Source: CAD feature listing. Evaluate the final solid. Frame: model axes, mm. Round coordinates to 2 decimals unless told otherwise and drop trailing zeros. Loops run counter-clockwise (first coordinate to the right, second up) from the corner with the lowest first, then second, coordinate; pieces in that order, holes last. Notation, with made-up numbers: M -7,78.25 L 30,78.25 A11 cw 30,95.25 Z; hole C 13,57.5 d6. An arc over 180 degrees is marked long. Write each question's results on one line, items separated by ' | '. Start each with the question number.
1. Section B-B on y = -15. Output: boundary loops of the cut face in (x, z).
2. Ray query, line 1 (X direction, y = -3.5, z = -84.5); line 2 (X direction, y = -3, z = -99.5); line 3 (X direction, y = -3, z = -218.5). Return the intervals inside material, ascending.
3. Section A-A on z = -59. Output: boundary loops of the cut face in (x, y).
4. Contact query for flat-ended pins moving along their axis: pin 1 Ø10 at (x, y) = (641.5, -14) entering from +Z; pin 2 Ø1 at (x, y) = (671, -17) entering from +Z; pin 3 Ø10 at (y, z) = (8, -150) entering from -X. Output: stop coordinate, or through.
from build123d import *

# Parameters (mm, degrees)
F0_R     = 25
F1_DEPTH = 1000
F2_R     = 5
F3_DEPTH = 50
F4_R     = 5
F5_DEPTH = 200
F6_R     = 5
F7_DEPTH = 350
F8_R     = 5
F9_DEPTH = 280


with BuildPart() as f1:
    # F0 (on Right) → F1 (new body)
    with BuildSketch(Plane.YZ):
        with Locations((0, 53.862866)):
            Circle(F0_R)
    extrude(amount=F1_DEPTH)

    # F2 (on Top) → F3 (join)
    with BuildSketch(Plane.XY):
        with Locations((500, 0)):
            Circle(F2_R)
        with Locations((250, 0)):
            Circle(F2_R)
        with Locations((750, 0)):
            Circle(F2_R)
    extrude(amount=F3_DEPTH)

    # F4 (on face) → F5 (join)
    with BuildSketch(Plane(origin=(0, 0, 0), x_dir=(1, 0, 0), z_dir=(0, 0, -1))):
        with Locations((750, 0)):
            Circle(F4_R)
    extrude(amount=F5_DEPTH)

    # F6 (on face) → F7 (join)
    with BuildSketch(Plane(origin=(0, 0, 0), x_dir=(1, 0, 0), z_dir=(0, 0, -1))):
        with Locations((500, 0)):
            Circle(F6_R)
    extrude(amount=F7_DEPTH)

    # F8 (on face) → F9 (join)
    with BuildSketch(Plane(origin=(0, 0, 0), x_dir=(1, 0, 0), z_dir=(0, 0, -1))):
        with Locations((250, 0)):
            Circle(F8_R)
    extrude(amount=F9_DEPTH)


solid = f1.part
Taken from the geometry:
1) outline: M 0,33.86 L 1000,33.86 L 1000,73.86 L 0,73.86 Z
2) line 1: 246.43 to 253.57, 496.43 to 503.57, 746.43 to 753.57 | line 2: 246 to 254, 496 to 504, 746 to 754 | line 3: 246 to 254, 496 to 504
3) outline: C 250,0 d10; C 500,0 d10; C 750,0 d10
4) pin 1: z = 77.19 | pin 2: z = 72.64 | pin 3: x = 246
